Geometry: see drawing. Coordinates: mm, zero at the bounding-box minimum. A direction names the side the tool comes from. Coordinates: 2 decimals unless noted, no trailing zeros. Order: outer loops, then holes, each group sorted by start corner. A loop starts at its lowest first (then second) coordinate and runs counter-clockwise, first axis right, second up. Notation, with made-up numbers: M 48.25,38 L 94.25,38 A27 cw 94.25,76 Z; hole C 62,77 d6. An arc over 180 degrees is marked long. One line per item, written item: value.
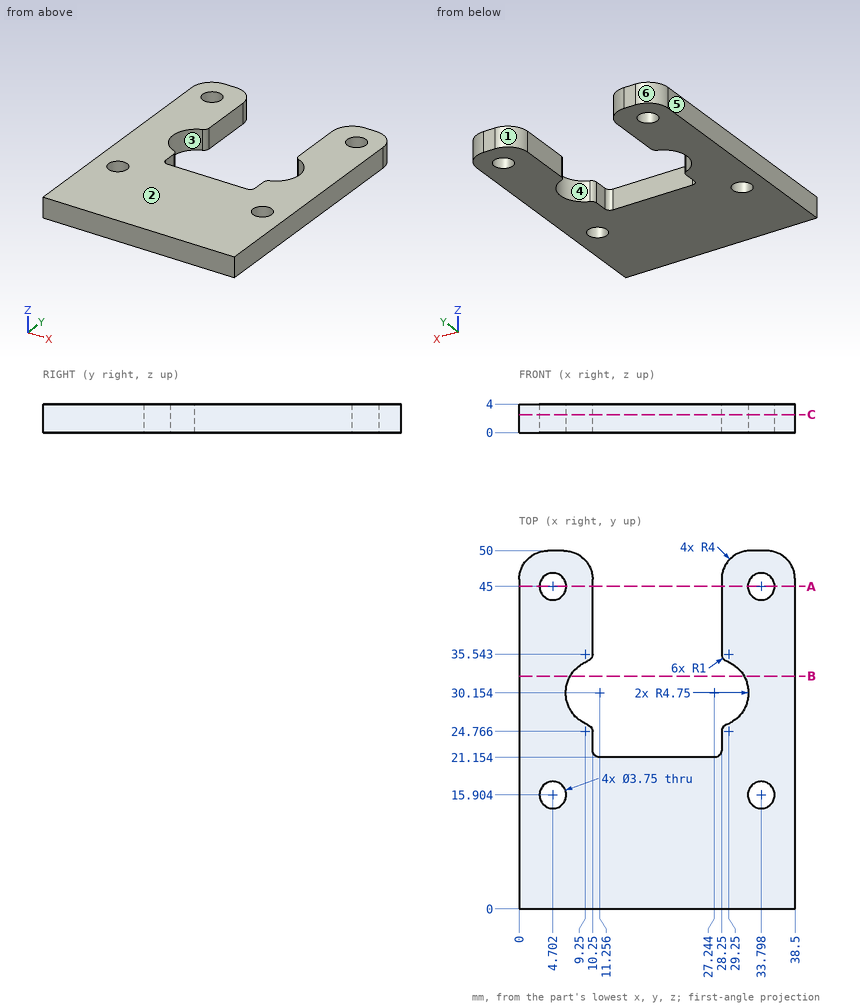
(1) Cut plane B-B on y = 32.5. Output: boundary loops of the cut face in (x, z) (1 decimal).
Data:
outline: M 0,0 L 7.1,0 L 7.1,4 L 0,4 Z; M 31.4,0 L 38.5,0 L 38.5,4 L 31.4,4 Z
(2) Draft query along Y for the marked faces 3, 4, 5 and 6. Return one class per face: released by +Y, released by -Y, zero draft, split by the parting line, or undercut.
Data:
face 3: undercut
face 4: undercut
face 5: zero draft
face 6: released by +Y
(3) Cut plane C-C on z = 2.5. Give the number of separate pieces and of enclosed holes in the cut face, plus the area to 3 significant figures.
Data:
separate pieces: 1
enclosed holes: 4
area: 1,300 mm2
(4) Cut plane A-A on y = 45. Output: boundary loops of the cut face in (x, z).
Data:
outline: M 0,0 L 2.83,0 L 2.83,4 L 0,4 Z; M 6.58,0 L 10.25,0 L 10.25,4 L 6.58,4 Z; M 28.25,0 L 31.92,0 L 31.92,4 L 28.25,4 Z; M 35.67,0 L 38.5,0 L 38.5,4 L 35.67,4 Z
(5) First-contact query: pin 1 (1.5 mm diameter, centred on x = 15, z = 2, fed in from +Y). Flat tip, straight axial feed; report the tip coordinate or a pass-through.
Data:
pin 1: stops at y = 21.15
(6) Access query for the marked faces 1 and 2. Directions: +Z, -Z, +X, -X, +Y, -Y. A direction counts if a zero-diameter tool reaches every point of the face in a straight line with its end or side. Return the directions, or none.
Data:
face 1: +Z, -Z, +Y
face 2: +Z, +X, -X, +Y, -Y
(7) Ray query, line 1 (X direction, y = 39, z = 0.95); line 2 (X direction, y = 15.5, z = 3.6); line 3 (X direction, y = 28.5, z = 2.2) (1 decimal). Return the intervals inside material, ascending. Write a range as from..to.
Data:
line 1: x = 0..10.25, 28.25..38.5
line 2: x = 0..2.87, 6.53..31.97, 35.63..38.5
line 3: x = 0..6.8, 31.7..38.5
